Source: three-view drawing plus pictorial views. Frame: mm from the lowest corner of the part. Give positions to 0.01 mm unless a question says otherwise; leave off trailing zeros. Loops run counter-clockwise (first coordinate to the right, second up) from the corner with the lowest first, then second, coordinate; pieces in that order, holes last. Notation, with made-up numbers: (65, 84.5) -> (92, 84.5) arc R22 ccw to (92, 95.5) -> close; hole circle Ø9 at (16.25, 21.5). An arc over 180 degrees is marked (long way). Answer as a JSON object with one key per item and string values. Group by question number.
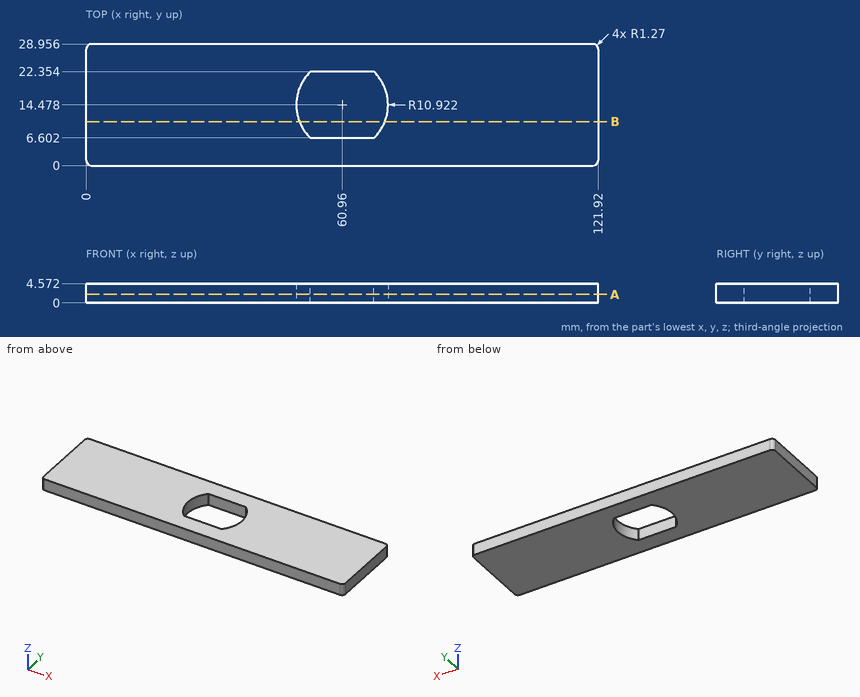
(1) Section query A-A on z = 2. Return the cut outline in (x, y).
(2) Material intervals for line 1 (Y direction, x = 62.5, z = 4.2); line 2 (X direction, y = 13.75, z = 1.15); line 3 (X direction, y = 13.5, z = 2.9), sorted ascending. Write a range as from..to.
(3) Section query B-B on y = 10.5. Return the cut outline in (x, z), plus the area to 3 significant figures.
Result:
{
 "1": {"outline": "(0, 1.27) arc R1.27 ccw to (1.27, 0) -> (120.65, 0) arc R1.27 ccw to (121.92, 1.27) -> (121.92, 27.69) arc R1.27 ccw to (120.65, 28.96) -> (1.27, 28.96) arc R1.27 ccw to (0, 27.69) -> close; hole (53.39, 6.6) -> (68.53, 6.6) arc R10.92 ccw to (68.53, 22.35) -> (53.39, 22.35) arc R10.92 ccw to start"},
 "2": {"line 1": "0..6.6, 22.35..28.96", "line 2": "0..50.06, 71.86..121.92", "line 3": "0..50.08, 71.84..121.92"},
 "3": {"outline": "(0, 0) -> (50.79, 0) -> (50.79, 4.57) -> (0, 4.57) -> close; (71.13, 0) -> (121.92, 0) -> (121.92, 4.57) -> (71.13, 4.57) -> close", "area": "464 mm²"}
}
